Could you check a few things on this model? Use its own coordinates, in mm. Face numbers are marked on the shaded views. A direction names the side the tool comes from. Round coordinates to 2 decimals unless told otherwise and drop trailing zeros. Write each loop counter-clockwise with the first axis right and the second up, starting at its lowest first coordinate (ties: lowest second). Pieces come first, ordered by that corner, then holes. Notation, with made-up numbers: (59.5, 47) -> (72.5, 47) arc R16 ccw to (72.5, 76) -> close; hole circle Ø11 at (-29.75, 80). An arc over 180 degrees is marked (long way). One line per question, with ' | ' between items. Start each with the question number.
1. Imagine slicing it at D-D, the plane x = -8.75. List the corners of the cut face in (y, z) for me, and give its area (3 significant figures).
2. For the marked faces 1 and 2, which set-ups out of +Z, -Z, +X, -X, +Y, -Y let a thin tool reach every point of the face, with its end or its side?
3. For pin 1 Ø3 at (x, z) = (-8.5, -32) entering from +Y; pin 2 Ø1.5 at (x, z) = (3.5, -30) entering from +Y; pin 3 Ø1 at (y, z) = (-9, -14.5) entering from +X, each with a flat end and sliding along its axis, tell me the tip position at first contact or that it passes through.
4. Imagine slicing it at A-A, the plane x = -4.5. List the corners of the cut face in (y, z) for me.
5. If I drill on line 1 along Y through (x, z) = (0, -38.7); line 2 along X through (y, z) = (-9.5, -12); line 3 along Z through (x, y) = (0.5, -10.5), over which ranges is the centre line in solid material (lowest first)? Write a range as [from, to].
6. Imagine slicing it at C-C, the plane y = -2.5. List the corners of the cut face in (x, z) for me, and give its area (3 significant figures).
7. Thinking about a two-plate mould opening in X: for the marked faces 3, 4 and 5, which applies, released by +X, released by -X, zero draft, split by the parting line, or undercut?
8. Imagine slicing it at B-B, the plane z = -27. List the corners of the cut face in (x, y) for me, and give its area (3 significant figures).
from build123d import *

# Parameters (mm, degrees)
F1_R     = 13
F2_DEPTH = 41
F3_DEPTH = 38
F4_R     = 7.5
F5_DEPTH = 25


with BuildPart() as f2:
    # F1 (on Top) → F2 (new body)
    with BuildSketch(Plane.XY):
        Circle(F1_R)
    extrude(amount=-F2_DEPTH)

    # F0 (on Top) → F3 (cut)
    with BuildSketch(Plane.XY):
        Polygon((-0.524238, 11.072722), (-9.851377, 5.082358), (-9.32714, -5.990364), (0.524238, -11.072722), (9.851377, -5.082358), (9.32714, 5.990364), align=None)
    extrude(amount=-F3_DEPTH, mode=Mode.SUBTRACT)

    # F4 (on face) → F5 (cut)
    with BuildSketch(Plane(origin=(0, 0, -41), x_dir=(1, 0, 0), z_dir=(0, 0, -1))):
        Circle(F4_R)
    extrude(amount=-F5_DEPTH, mode=Mode.SUBTRACT)


solid = f2.part
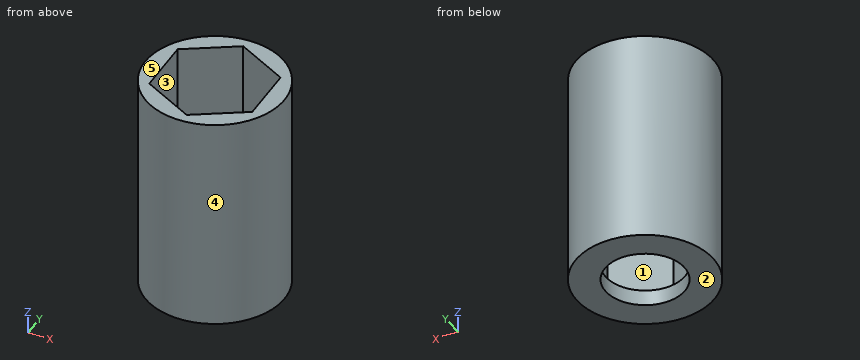
Geometry results:
1) outline: (-9.61, -41) -> (9.61, -41) -> (9.61, 0) -> (5.79, 0) -> (5.79, -38) -> (-6.29, -38) -> (-6.29, 0) -> (-9.61, 0) -> close | area: 329 mm2
2) face 1: +Z | face 2: -Z, +X, -X, +Y, -Y
3) pin 1: stops at y = 10.95 | pin 2: stops at y = 12.71 | pin 3: stops at x = 9.84
4) outline: (-12.2, -41) -> (-6, -41) -> (-6, -38) -> (-8.48, -38) -> (-8.48, 0) -> (-12.2, 0) -> close; (6, -41) -> (12.2, -41) -> (12.2, 0) -> (8.52, 0) -> (8.52, -38) -> (6, -38) -> close
5) line 1: y = [-13, -7.5], [7.5, 13] | line 2: x = [-8.87, -2.52], [2.97, 8.87] | line 3: z = [-41, -38]
6) outline: (-12.76, -41) -> (-7.07, -41) -> (-7.07, -38) -> (-9.49, -38) -> (-9.49, 0) -> (-12.76, 0) -> close; (7.07, -41) -> (12.76, -41) -> (12.76, 0) -> (9.73, 0) -> (9.73, -38) -> (7.07, -38) -> close | area: 273 mm2
7) face 3: undercut | face 4: split by the parting line | face 5: zero draft
8) outline: circle Ø26 at (0, 0); hole (-9.85, 5.08) -> (-9.33, -5.99) -> (0.52, -11.07) -> (9.85, -5.08) -> (9.33, 5.99) -> (-0.52, 11.07) -> close | area: 212 mm2
